from build123d import *

# Parameters (mm, degrees)
BOSS_EXTRUDE1_DEPTH = 15
SKETCH3_R           = 2
CUT_EXTRUDE1_DEPTH  = 12.5
SKETCH4_W           = 25.9
SKETCH4_H           = 8
BOSS_EXTRUDE2_DEPTH = 20


with BuildPart() as part:
    # Sketch2 → Boss-Extrude1 (new body)
    with BuildSketch(Plane(origin=(0, 0, 0), x_dir=(1, 0, 0), z_dir=(0, 1, 0))):
        with BuildLine():
            Line((-30, -4), (0, -4))
            ThreePointArc((0, -4), (-4, 0), (0, 4))
            Line((0, 4), (-30, 4))
            Line((-30, 4), (-30, -4))
        make_face()
        with BuildLine():
            ThreePointArc((0, 4), (-4, 0), (0, -4))
            Line((0, -4), (0, 4))
        make_face()
        with BuildLine():
            Line((0, 4), (0, -4))
            ThreePointArc((0, -4), (2.828427125, -2.828427125), (4, 0))
            ThreePointArc((4, 0), (2.828427125, 2.828427125), (0, 4))
        make_face()
    extrude(amount=BOSS_EXTRUDE1_DEPTH)

    # Sketch3 → Cut-Extrude1 (cut)
    with BuildSketch(Plane(origin=(0, 15, 0), x_dir=(1, 0, 0), z_dir=(0, 1, 0))):
        with Locations(Location((0, 0, 0), (0, 0, 270))):
            Circle(SKETCH3_R)
    extrude(amount=-CUT_EXTRUDE1_DEPTH, mode=Mode.SUBTRACT)

    # Sketch4 → Boss-Extrude2 (add)
    with BuildSketch(Plane(origin=(0, 15, 0), x_dir=(1, 0, 0), z_dir=(0, 1, 0))):
        with Locations((-17.05, 0)):
            Rectangle(SKETCH4_W, SKETCH4_H)
    extrude(amount=BOSS_EXTRUDE2_DEPTH)


solid = part.part
Input: part model. Units: mm. Frame: model coordinates. A direction names the side the tool comes from. Coordinates: 2 decimals unless noted, no trailing zeros. Loops run counter-clockwise (first coordinate to the right, second up) from the corner with the lowest first, then second, coordinate; pieces in that order, holes last.
(1) Pull-direction query (X, two-part tool) for faces 1 (the face through (0, 2.5, 0)), 2 (the face through (-30, 17, 0)), 3 (the face through (-2, 15, -1)), 4 (the face through (-2, 9, 0)); classes: released by +X, released by -X, zero draft, split by the parting line, or undercut.
(2) Section D-D on y = 15.5. Return the cut outline in (x, z).
(3) Section C-C on z = 1.25. Return the cut outline in (x, y).
(4) Section B-B on x = 1.5. Return the cut outline in (y, z), then the cut area to 3 significant figures.
(5) Material intervals for probe 1 along X at (y, z) = (23, -0.25); probe 2 along Y at (x, z) = (0.5, 1.75); probe 3 along Y at (x, z) = (-3, -1.5), sorted ascending.
(6) First-contact query: pin 1 Ø4.5 at (x, z) = (0.5, -0.5) entering from +Y; pin 2 Ø3 at (y, z) = (20, 0) entering from +X; pin 3 Ø3.5 at (x, z) = (0, 0) entering from +Y. Flat tips, straight axial feed; report the tip coordinate or a pass-through.
(7) Section A-A on y = 12. Return the cut outline in (x, z).
(8) Set-up query: faces 5 (the face through (-4.1, 25, 0)), 6 (the face through (-15, 17, 4)). Return all of +Z, -Z, +X, -X, +Y, -Y with unobstructed straight access to the full face (end or side cutting, diameter ignored); none if empty.
Data:
1. face 1: undercut
1. face 2: released by -X
1. face 3: zero draft
1. face 4: undercut
2. outline: (-30, -4) - (-4.1, -4) - (-4.1, 4) - (-30, 4) - close
3. outline: (-30, 0) - (3.8, 0) - (3.8, 15) - (1.56, 15) - (1.56, 2.5) - (-1.56, 2.5) - (-1.56, 15) - (-4.1, 15) - (-4.1, 35) - (-30, 35) - close
4. outline: (0, -3.71) - (15, -3.71) - (15, -1.32) - (2.5, -1.32) - (2.5, 1.32) - (15, 1.32) - (15, 3.71) - (0, 3.71) - close
4. area: 78.2 mm2
5. probe 1: x = -30 to -4.1
5. probe 2: y = 0 to 2.5
5. probe 3: y = 0 to 15
6. pin 1: stops at y = 15
6. pin 2: stops at x = -4.1
6. pin 3: stops at y = 2.5
7. outline: (-30, -4) - (0, -4) arc R4 ccw to (0, 4) - (-30, 4) - close; hole circle Ø4 at (0, 0)
8. face 5: +Z, -Z, +X, +Y
8. face 6: +Z, +X, -X, +Y, -Y
